Can you work these out from the model? Positions are in its coordinate system, mm. Coordinates: 2 decimals unless noted, no trailing zeros. Write each loop counter-clockwise with the first axis right and the second up, starting at its lowest first coordinate (ties: lowest second). Pieces come first, ordered by that corner, then holes. Notation, with made-up numbers: (24, -32) -> (42, -32) arc R13 cw to (42, -27) -> close; hole circle Ø9 at (-4, -8). An arc over 180 degrees is marked (long way). Use one line per item in the form item = value.
```python
from build123d import *

# Parameters (mm, degrees)
SKETCH1_W                = 152.4
SKETCH1_H                = 152.4
BOSS_EXTRUDE1_DEPTH      = 9.525
F_5_16_18_TAPPED_HOLE1_D = 6.5278
F_5_16_CLEARANCE_HOLE1_D = 8.4328


with BuildPart() as part:
    # Sketch1 → Boss-Extrude1 (new body)
    with BuildSketch(Plane.XY):
        with Locations((76.2, 76.2)):
            Rectangle(SKETCH1_W, SKETCH1_H)
    extrude(amount=BOSS_EXTRUDE1_DEPTH)

    # 5/16-18 Tapped Hole1 (through all)
    with Locations(Plane.XY.offset(9.525)):
        with Locations((109.5375, 101.6), (42.8625, 101.6), (109.5375, 50.8), (42.8625, 50.8)):
            Hole(F_5_16_18_TAPPED_HOLE1_D / 2)

    # 5/16 Clearance Hole1 (through all)
    with Locations(Plane.XY.offset(9.525)):
        with Locations((95.25, 127), (57.15, 127), (95.25, 25.4), (57.15, 25.4)):
            Hole(F_5_16_CLEARANCE_HOLE1_D / 2)


solid = part.part
```
Q1. Suppose I cut it at C-C (z = 5). Give the number of separate pieces and of enclosed holes in the cut face, then the cut area to 3 significant figures.
Return value:
separate_pieces = 1
enclosed_holes = 8
area = 22,900 mm2
Q2. If I drill on line 1 (Y direction, x = 95.25, z = 6.75); line 2 (Y direction, x = 55.5, z = 5); line 3 (X direction, y = 24, z = 6.75), over which ranges is the centre line in solid material (lowest first)? Write a range as from..to.
Return value:
line_1 = 0..21.18, 29.62..122.78, 131.22..152.4
line_2 = 0..21.52, 29.28..123.12, 130.88..152.4
line_3 = 0..53.17, 61.13..91.27, 99.23..152.4
Q3. Suppose I cut it at A-A (x = 57.15). Write out the boundary of the cut face in (y, z) (3 decimals).
Return value:
outline = (0, 0) -> (21.184, 0) -> (21.184, 9.525) -> (0, 9.525) -> close; (29.616, 0) -> (122.784, 0) -> (122.784, 9.525) -> (29.616, 9.525) -> close; (131.216, 0) -> (152.4, 0) -> (152.4, 9.525) -> (131.216, 9.525) -> close
Q4. Suppose I cut it at B-B (y = 25.4). Write out the boundary of the cut face in (x, z) (3 decimals), then the cut area to 3 significant figures.
Return value:
outline = (0, 0) -> (52.934, 0) -> (52.934, 9.525) -> (0, 9.525) -> close; (61.366, 0) -> (91.034, 0) -> (91.034, 9.525) -> (61.366, 9.525) -> close; (99.466, 0) -> (152.4, 0) -> (152.4, 9.525) -> (99.466, 9.525) -> close
area = 1,290 mm2
Q5. Thinking about a two-plate mould opening in X: for faces 1 (the cylindrical face through (55.2, 123.26, 4.7)), 2 (the flat face through (0, 75, 5)), 3 (the flat face through (152.4, 75, 5)), 4 (the flat face through (75, 0, 5)), which applies, released by +X, released by -X, zero draft, split by the parting line, or undercut?
Return value:
face_1 = undercut
face_2 = released by -X
face_3 = released by +X
face_4 = zero draft
